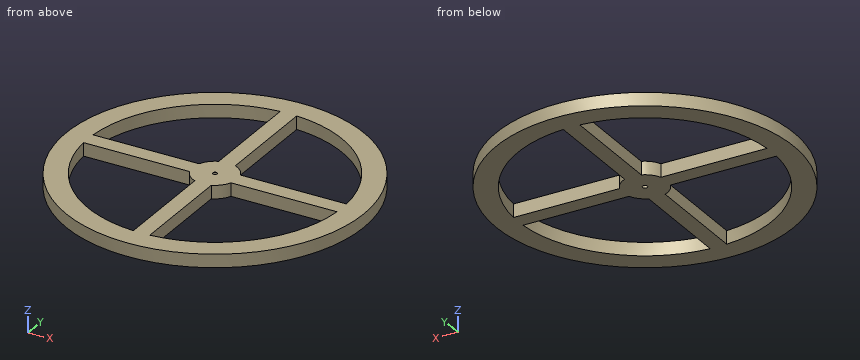
from build123d import *

# Parameters (mm, degrees)
SKETCH1_R           = 45
BOSS_EXTRUDE1_DEPTH = 4
CUT_EXTRUDE1_DEPTH  = 64.765194268


# Read off the part's stored shape, not the designer's step: Cavity1
with BuildPart() as part:
    # Sketch1 → Boss-Extrude1 (new body)
    with BuildSketch(Plane.XY):
        Circle(SKETCH1_R)
    extrude(amount=BOSS_EXTRUDE1_DEPTH)

    # Cavity1 outline → Cavity1 (revolve, cut)
    with BuildSketch(Plane.XZ):
        Polygon((0.75, 0), (0.75, 3.9), (0.65, 4), (0, 4), (0, 0), align=None)
    revolve(axis=Axis((0, 0, 0), (0, 0, 1)), mode=Mode.SUBTRACT)

    # Sketch2 → Cut-Extrude1 (cut, through all)
    with BuildSketch(Plane.XY.offset(4)):
        with BuildLine():
            Line((2.5, 6.241391614), (2.5, 38.313254027))
            ThreePointArc((2.5, 38.313254027), (27.149175256, 27.149175256), (38.313254027, 2.5))
            Line((38.313254027, 2.5), (6.241391614, 2.5))
            ThreePointArc((6.241391614, 2.5), (4.754207047, 4.754207047), (2.5, 6.241391614))
        make_face()
        with BuildLine():
            Line((-2.5, -38.313254027), (-2.5, -6.241391614))
            ThreePointArc((-2.5, -6.241391614), (-4.754207047, -4.754207047), (-6.241391614, -2.5))
            Line((-6.241391614, -2.5), (-38.313254027, -2.5))
            ThreePointArc((-38.313254027, -2.5), (-27.149175256, -27.149175256), (-2.5, -38.313254027))
        make_face()
        with BuildLine():
            Line((2.5, -38.313254027), (2.5, -6.241391614))
            ThreePointArc((2.5, -6.241391614), (4.754207047, -4.754207047), (6.241391614, -2.5))
            Line((6.241391614, -2.5), (38.313254027, -2.5))
            ThreePointArc((38.313254027, -2.5), (27.149175256, -27.149175256), (2.5, -38.313254027))
        make_face()
        with BuildLine():
            Line((-2.5, 6.241391614), (-2.5, 38.313254027))
            ThreePointArc((-2.5, 38.313254027), (-27.149175256, 27.149175256), (-38.313254027, 2.5))
            Line((-38.313254027, 2.5), (-6.241391614, 2.5))
            ThreePointArc((-6.241391614, 2.5), (-4.754207047, 4.754207047), (-2.5, 6.241391614))
        make_face()
    extrude(amount=-CUT_EXTRUDE1_DEPTH, mode=Mode.SUBTRACT)


solid = part.part
The listing builds one solid part. Answer for the finished solid, in the listing's coordinates (mm). Give positions to 0.01 mm unless a question says otherwise; leave off trailing zeros. Loops run counter-clockwise (first coordinate to the right, second up) from the corner with the lowest first, then second, coordinate; pieces in that order, holes last. Notation, with made-up numbers: (-19, 80.25) - (-9, 80.25) arc R16 ccw to (-9, 103.25) - close; hole circle Ø5 at (41, 28). An arc over 180 degrees is marked (long way). Answer as a JSON object with one key per item and string values.
1. Flat-ended cylindrical pins translate along their axes: pin 1 Ø1.2 at (x, z) = (-26, 2) entering from -Y; pin 2 Ø1.2 at (y, z) = (-24, 2) entering from -X; pin 3 Ø1.2 at (y, z) = (19, 2) entering from +X; pin 4 Ø6 at (x, y) = (33, 6) entering from -Z. Find the tip coordinate at first contact, or state that the pin passes through.
Determined:
{"pin 1": "y = -37.15", "pin 2": "x = -38.44", "pin 3": "x = 41.07", "pin 4": "through"}
2. A cutting plane is placed at C-C (y = -26). Write down the section's boundary in (x, z), then the cut area to 3 significant figures.
Determined:
{"outline": "(-36.73, 0) - (-28.25, 0) - (-28.25, 4) - (-36.73, 4) - close; (-2.5, 0) - (2.5, 0) - (2.5, 4) - (-2.5, 4) - close; (28.25, 0) - (36.73, 0) - (36.73, 4) - (28.25, 4) - close", "area": "87.8 mm²"}
3. Find the intervals of material crossed by L1, parallel to Y at x = 0, z = 1.8; L2, parallel to Y at x = -28, z = 2.6; L3, parallel to X at y = 11, z = 2.15, in increasing order. Write a range as [from, to].
Determined:
{"L1": "[-45, -0.75], [0.75, 45]", "L2": "[-35.23, -26.27], [-2.5, 2.5], [26.27, 35.23]", "L3": "[-43.63, -36.79], [-2.5, 2.5], [36.79, 43.63]"}
4. A cutting plane is placed at B-B (x = -30). Write down the section's boundary in (y, z), then the cut area to 3 significant figures.
Determined:
{"outline": "(-33.54, 0) - (-23.96, 0) - (-23.96, 4) - (-33.54, 4) - close; (-2.5, 0) - (2.5, 0) - (2.5, 4) - (-2.5, 4) - close; (23.96, 0) - (33.54, 0) - (33.54, 4) - (23.96, 4) - close", "area": "96.6 mm²"}
5. A cutting plane is placed at A-A (z = 2.7). Write down the section's boundary in (x, y).
Determined:
{"outline": "circle Ø90 at (0, 0); hole (-38.31, -2.5) arc R38.39 ccw to (-2.5, -38.31) - (-2.5, -6.24) arc R6.72 cw to (-6.24, -2.5) - close; hole (-38.31, 2.5) - (-6.24, 2.5) arc R6.72 cw to (-2.5, 6.24) - (-2.5, 38.31) arc R38.39 ccw to start; hole circle Ø1.5 at (0, 0); hole (2.5, -38.31) arc R38.39 ccw to (38.31, -2.5) - (6.24, -2.5) arc R6.72 cw to (2.5, -6.24) - close; hole (2.5, 6.24) arc R6.72 cw to (6.24, 2.5) - (38.31, 2.5) arc R38.39 ccw to (2.5, 38.31) - close"}
